Read the model definition and answer for the solid it produces. Units are mm, in the model's axes. Round coordinates to 2 decimals unless told otherwise and drop trailing zeros. Order: outer loops, then holes, each group sorted by start corner. A loop starts at its lowest first (then second) coordinate and runs counter-clockwise, first axis right, second up. Notation, with made-up numbers: (-21, 27.25) - (22, 27.25) arc R10 ccw to (22, 42.25) - close; hole circle Ø2 at (19.25, 53.25). An arc over 180 degrees is marked (long way). Put each result on its own line as item: value. Start each with the question number.
Q1. Section B-B on y = 283 is taken. Give the vertices of the cut face in (x, z), then the cut area to 3 significant figures.
Q2. Find the intervals of material crossed by line 1 along Y through (x, z) = (-100, 115); line 2 along Z through (x, y) = (-81, 238); line 3 along Z through (x, y) = (-29, 230), in increasing order. Write a range as from..to.
Q3. Section A-A on z = 58 is taken. Give the vertices of the cut face in (x, y), then the cut area to 3 significant figures.
Q4. For a pull along Z with two mould halves and no side action, classify faces 1 (the face through (-57, 210, 169.105)), 2 (the face through (-55.38, 297.82, 57.75)), 3 (the face through (-112.34, 162, 83)) as pulls with the +Z half, pulls with the -Z half, needs draft (parallel to the pull), parting line crosses it, or undercut.
Q5. Section C-C on x = -99.5 is taken. Give the vertices of the cut face in (y, z).
from build123d import *

# Parameters (mm, degrees)
F0_W     = 112.340003252
F0_H     = 169.1052764654
F2_DEPTH = 425.2858813852
F3_R     = 61.9097520686
F4_DEPTH = 148.8002743572
F5_SIZE  = 5.08


with BuildPart() as f2:
    # F0 (on Front) → F2 (new body)
    with BuildSketch(Plane.XZ):
        with Locations((-56.170001626, 84.5526382327)):
            Rectangle(F0_W, F0_H)
    extrude(amount=-F2_DEPTH)

    # F3 (on face) → F4 (cut)
    with BuildSketch(Plane.YZ):
        with Locations((240.6340688467, 81.4660638571)):
            Circle(F3_R)
    extrude(amount=-F4_DEPTH, mode=Mode.SUBTRACT)

    # F5
    f5_edges = [f2.edges().sort_by_distance(p)[0] for p in [
        (-56.170002, 425.285881, 169.105276),
        (-56.170002, 0, 169.105276),
        (-56.170002, 0, 0),
    ]]
    chamfer(f5_edges, length=F5_SIZE)


solid = f2.part
Findings:
1. outline: (-112.34, 0) - (0, 0) - (0, 36.32) - (-112.34, 36.32) - close; (-112.34, 126.61) - (0, 126.61) - (0, 169.11) - (-112.34, 169.11) - close
1. area: 8,850 mm2
2. line 1: 0..188.59, 292.68..425.29
2. line 2: 0..19.61, 143.32..169.11
2. line 3: 0..20.48, 142.46..169.11
3. outline: (-112.34, 0) - (0, 0) - (0, 183.34) - (-112.34, 183.34) - close; (-112.34, 297.92) - (0, 297.92) - (0, 425.29) - (-112.34, 425.29) - close
3. area: 34,900 mm2
4. face 1: pulls with the +Z half
4. face 2: undercut
4. face 3: needs draft
5. outline: (0, 5.08) - (5.08, 0) - (425.29, 0) - (425.29, 164.03) - (420.21, 169.11) - (5.08, 169.11) - (0, 164.03) - close; hole circle Ø123.82 at (240.63, 81.47)
